Build history of the part. All positions in model axes, mm. A direction names the side the tool comes from. Give positions to 0.01 mm unless a question says otherwise; leave off trailing zeros. Write each loop counter-clockwise with the first axis right and the second up, starting at its lowest first coordinate (ties: lowest second). Pieces come first, ordered by that corner, then holes.
from build123d import *

# Parameters (mm, degrees)
F0_R     = 25.4
F0_R_2   = 12.7
F1_DEPTH = 25.4
F2_DEPTH = 88.392
F3_DEPTH = 51.308
F4_R     = 12.7


with BuildPart() as f1:
    # F0 (on Top) → F1 (new body)
    with BuildSketch(Plane.XY):
        with BuildLine():
            ThreePointArc((14.569248, -48.665974), (40.747747, -30.335805), (50.8, 0))
            ThreePointArc((50.8, 0), (40.747747, 30.335805), (14.569248, 48.665974))
            ThreePointArc((14.569248, 48.665974), (-50.8, 0), (14.569248, -48.665974))
        make_face()
        Circle(F0_R, mode=Mode.SUBTRACT)
        with BuildLine():
            ThreePointArc((14.569248, 48.665974), (40.747747, 30.335805), (50.8, 0))
            ThreePointArc((50.8, 0), (40.747747, -30.335805), (14.569248, -48.665974))
            Line((14.569248, -48.665974), (95.849248, -24.332987))
            ThreePointArc((95.849248, -24.332987), (63.164624, 0), (95.849248, 24.332987))
            Line((95.849248, 24.332987), (14.569248, 48.665974))
        make_face()
        with BuildLine():
            ThreePointArc((113.964624, 0), (108.938498, 15.167903), (95.849248, 24.332987))
            ThreePointArc((95.849248, 24.332987), (63.164624, 0), (95.849248, -24.332987))
            ThreePointArc((95.849248, -24.332987), (108.938498, -15.167903), (113.964624, 0))
        make_face()
        with Locations((88.564624, 0)):
            Circle(F0_R_2, mode=Mode.SUBTRACT)
    extrude(amount=F1_DEPTH)

    # F0 (on Top) → F2 (join)
    with BuildSketch(Plane.XY):
        with BuildLine():
            ThreePointArc((14.569248, -48.665974), (40.747747, -30.335805), (50.8, 0))
            ThreePointArc((50.8, 0), (40.747747, 30.335805), (14.569248, 48.665974))
            ThreePointArc((14.569248, 48.665974), (-50.8, 0), (14.569248, -48.665974))
        make_face()
        Circle(F0_R, mode=Mode.SUBTRACT)
    extrude(amount=F2_DEPTH)

    # F0 (on Top) → F3 (join)
    with BuildSketch(Plane.XY):
        with BuildLine():
            ThreePointArc((14.569248, 48.665974), (40.747747, 30.335805), (50.8, 0))
            ThreePointArc((50.8, 0), (40.747747, -30.335805), (14.569248, -48.665974))
            Line((14.569248, -48.665974), (95.849248, -24.332987))
            ThreePointArc((95.849248, -24.332987), (63.164624, 0), (95.849248, 24.332987))
            Line((95.849248, 24.332987), (14.569248, 48.665974))
        make_face()
    extrude(amount=F3_DEPTH)

    # F4
    f4_edges = [f1.edges().sort_by_distance(p)[0] for p in [
        (95.849248, -24.332987, 38.354),
        (95.849248, 24.332987, 38.354),
    ]]
    fillet(f4_edges, radius=F4_R)


solid = f1.part
1. Drill centre lines: line 1 along Y through (x, z) = (0, 44); line 2 along Y through (x, z) = (-22, 59); line 3 along Z through (x, y) = (101, 12). Where is each one in solid material? Low to high.
2. Mould opens along X. For faces 3 (the face through (-5.506, -24.796, 43.577)), 4 (the face through (69.776, -26.68, 38.535)), 5 (the face through (-23.3, -10.6, 88.392)) say: pulls with the +X half, pulls with the -X half, needs draft (parallel to the pull), parting line crosses it, or undercut.
3. Saw through at D-D on y = 5.5. Give the cut face in (x, z), plus the area to 3 significant figures.
4. 3-axis set-ups, long thin cutter, end or side, ignore diameter. For faces 1 (the face through (63.166, -0.224, 38.173)), 2 (the face through (30, 1, 0)): which of +Z, -Z, +X, -X, +Y, -Y reach the whole face in a straight line?
5. Saw through at C-C on z = 39.5. Give the cut face in (x, y) (1 decimal), plus the area to 3 significant figures.
6. Saw through at B-B on x = 0. Give the cut face in (y, z), plus the area to 3 significant figures.
7. Saw through at A-A on y = 20. Give the cut face in (x, z), plus the area to 3 significant figures.
8. Drop flat-ended pins along their axis: pin 1 (1 mm diameter, centred on x = 4.5, z = 21, fed in from -Y); pin 2 (3 mm diameter, centred on y = -26, z = 10.5, fed in from -X); pin 3 (8 mm diameter, centred on y = 14.5, z = 41.5, fed in from +X). Give the stop position or say it passes through.
Outcome:
1. line 1: y = -50.8 to -25.4, 25.4 to 50.8
1. line 2: y = -45.79 to -12.69, 12.69 to 45.79
1. line 3: z = 0 to 25.4
2. face 3: undercut
2. face 4: pulls with the +X half
2. face 5: needs draft
3. outline: (-50.5, 0) - (-24.8, 0) - (-24.8, 88.39) - (-50.5, 88.39) - close; (24.8, 0) - (77.12, 0) - (77.12, 25.4) - (63.77, 25.4) - (63.77, 51.31) - (50.5, 51.31) - (50.5, 88.39) - (24.8, 88.39) - close; (100.01, 0) - (113.36, 0) - (113.36, 25.4) - (100.01, 25.4) - close
3. area: 5,900 mm2
4. face 1: +Z, +X
4. face 2: -Z, +X, -X, +Y, -Y
5. outline: (14.6, -48.7) - (61.4, -34.6) arc R12.7 ccw to (68.1, -15) arc R25.4 cw to (68.1, 15) arc R12.7 ccw to (61.4, 34.6) - (14.6, 48.7) arc R50.8 ccw (long way) to start; hole circle Ø50.8 at (0, 0)
5. area: 7,780 mm2
6. outline: (-50.8, 0) - (-25.4, 0) - (-25.4, 88.39) - (-50.8, 88.39) - close; (25.4, 0) - (50.8, 0) - (50.8, 88.39) - (25.4, 88.39) - close
6. area: 4,490 mm2
7. outline: (-46.7, 0) - (-15.66, 0) - (-15.66, 88.39) - (-46.7, 88.39) - close; (15.66, 0) - (104.22, 0) - (104.22, 25.4) - (70.25, 25.4) - (70.25, 51.31) - (46.7, 51.31) - (46.7, 88.39) - (15.66, 88.39) - close
7. area: 7,560 mm2
8. pin 1: stops at y = -50.64
8. pin 2: stops at x = -44.5
8. pin 3: stops at x = 69.86
